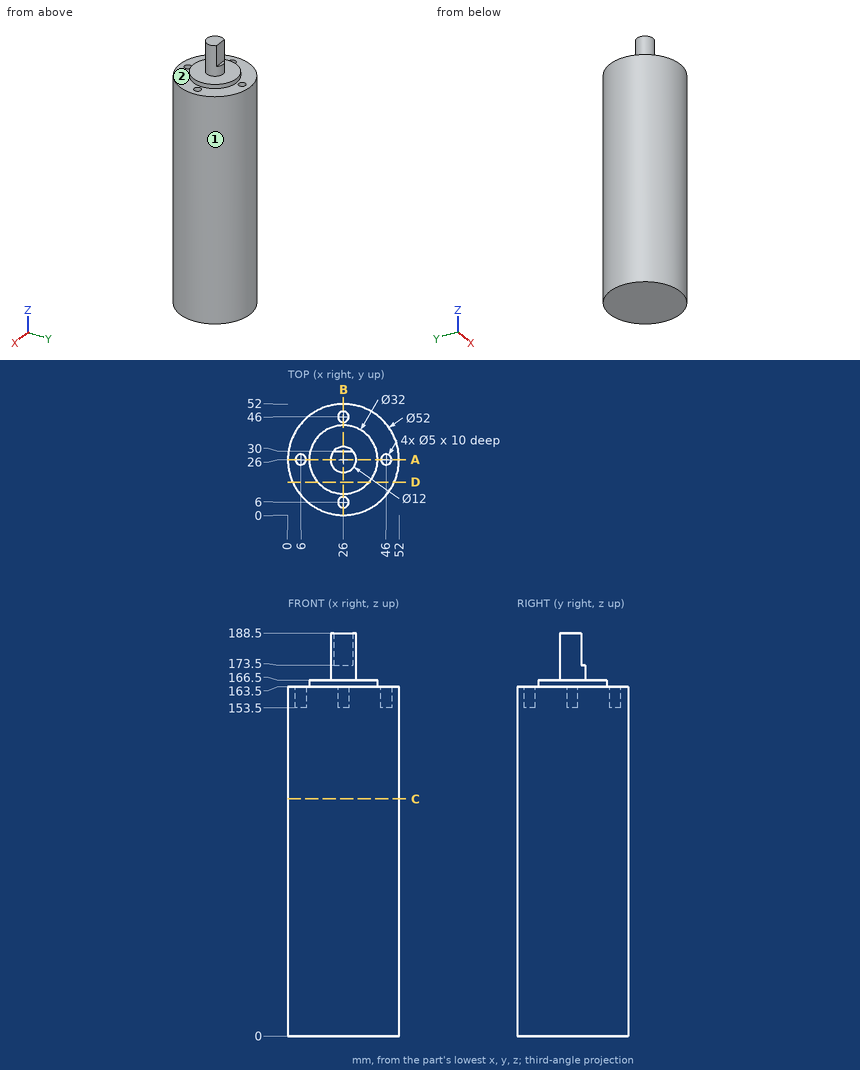
Answer from the drawing. Dimensions are ordinates in mm from the lowest x, y and z of the part. A direction names the side the tool comes from. Coordinates: 2 decimals unless noted, no trailing zeros. Loops run counter-clockwise (first coordinate to the right, second up) from the corner with the lowest first, then second, coordinate; pieces in that order, holes last.
1) Section A-A (y = 26) is taken. Give the vertices of the cut face in (x, z).
Results:
outline: (0, 0) - (52, 0) - (52, 163.5) - (48.5, 163.5) - (48.5, 153.5) - (43.5, 153.5) - (43.5, 163.5) - (42, 163.5) - (42, 166.5) - (32, 166.5) - (32, 188.5) - (20, 188.5) - (20, 166.5) - (10, 166.5) - (10, 163.5) - (8.5, 163.5) - (8.5, 153.5) - (3.5, 153.5) - (3.5, 163.5) - (0, 163.5) - close
2) Section B-B (x = 26) is taken. Give the vertices of the cut face in (y, z).
Results:
outline: (0, 0) - (52, 0) - (52, 163.5) - (48.5, 163.5) - (48.5, 153.5) - (43.5, 153.5) - (43.5, 163.5) - (42, 163.5) - (42, 166.5) - (32, 166.5) - (32, 173.5) - (30, 173.5) - (30, 188.5) - (20, 188.5) - (20, 166.5) - (10, 166.5) - (10, 163.5) - (8.5, 163.5) - (8.5, 153.5) - (3.5, 153.5) - (3.5, 163.5) - (0, 163.5) - close
3) Flat-ended cylindrical pins translate along their axes: pin 1 (2.5 mm diameter, centred on x = 27, y = 46, fed in from +Z); pin 2 (5 mm diameter, centred on y = 11.5, z = 104.5, fed in from +X); pin 3 (6 mm diameter, centred on x = 34, z = 128, fed in from +Y); pin 4 (6 mm diameter, centred on x = 46, y = 26, fed in from -Z). Find the tip coordinate at first contact, or state that the pin passes through.
Results:
pin 1: stops at z = 153.5
pin 2: stops at x = 49.07
pin 3: stops at y = 51.51
pin 4: stops at z = 0
4) Section C-C (z = 111) is taken. Give the vertices of the cut face in (x, y), plus the area to 3 significant figures.
Results:
outline: circle Ø52 at (26, 26)
area: 2,120 mm2
5) Section D-D (y = 15.5) is taken. Give the vertices of the cut face in (x, z).
Results:
outline: (2.21, 0) - (49.79, 0) - (49.79, 163.5) - (38.07, 163.5) - (38.07, 166.5) - (13.93, 166.5) - (13.93, 163.5) - (2.21, 163.5) - close
6) Consider probe 1 along Y at (x, z) = (26, 161); probe 2 along Y at (x, z) = (46, 158); probe 3 along Z at (x, y) = (33, 3.5). Determine where each line is inside the solid, lowest interval first.
Results:
probe 1: y = 0 to 3.5, 8.5 to 43.5, 48.5 to 52
probe 2: y = 9.39 to 23.5, 28.5 to 42.61
probe 3: z = 0 to 163.5
7) For the marked faces 1 and 2, determine the directions among +Z, -Z, +X, -X, +Y, -Y from which every point of the face is accessible in a straight line to the end or side of a thin tool.
Results:
face 1: +Z, -Z
face 2: +Z
